Verification items for the finished model (mm, model axes). Coordinates: 2 decimals unless noted, no trailing zeros. Loops run counter-clockwise (first coordinate to the right, second up) from the corner with the lowest first, then second, coordinate; pieces in that order, holes last. Notation, with made-up numbers: (54, -36.5) - (73, -36.5) arc R21 cw to (73, -30.5) - close; hole circle Ø8 at (33.5, 75.5). An arc over 180 degrees is marked (long way). One line per item, written item: value. Start each with the question number.
(1) Section check B-B (y = -33.5). Record the boundary of the cut face in (x, z), plus the area to 3 significant figures.
(2) Section check D-D (z = 34). Record the boundary of the cut face in (x, y).
(3) Section check C-C (x = 2.5). Record the boundary of the cut face in (y, z), plus the area to 3 significant figures.
(4) Thickness scan on probe 1 along Y at (x, z) = (4.3, -25); probe 2 along Y at (x, z) = (4.9, -21.5); probe 3 along Z at (x, y) = (2.5, 9). Record the ranges inside material, lowest first. Write a range as [from, to].
(5) Gauge pin test, flat ends, axial feed: P1, Ø3, axis at x = 4.5, y = -2.5, coming from the +Z side; P2, Ø8, axis at y = -30, z = 50, coming from the -X side. Record the tip position at first contact, or that the pin passes through.
(6) Section check A-A (z = -48). Record the boundary of the cut face in (x, y).
```python
from build123d import *

# Parameters (mm, degrees)
SKETCH1_R           = 5
SKETCH1_R_2         = 2.5
SKETCH1_W           = 10
SKETCH1_H           = 6
SKETCH1_W_2         = 20
BOSS_EXTRUDE1_DEPTH = 6
FILLET1_R           = 5
FILLET2_R           = 1


with BuildPart() as part:
    # Sketch1 → Boss-Extrude1 (new body)
    with BuildSketch(Plane(origin=(0, 0, 0), x_dir=(0, 0, -1), z_dir=(1, 0, 0))):
        with BuildLine():
            Line((0, 5), (65, 5))
            Line((65, 5), (65, 15))
            Line((65, 15), (-35, 15))
            Line((-35, 15), (-62, -21))
            ThreePointArc((-62, -21), (-64.112397745, -35.083328622), (-53.504672381, -44.584830184))
            Line((-53.504672381, -44.584830184), (-6, -56))
            Line((-6, -56), (65, -56))
            Line((65, -56), (65, -44))
            Line((65, -44), (0, -44))
            Line((0, -44), (0, 5))
        make_face()
        with Locations((-50, -30)):
            Circle(SKETCH1_R, mode=Mode.SUBTRACT)
        with Locations((55, 10)):
            Circle(SKETCH1_R_2, mode=Mode.SUBTRACT)
        with Locations((25, 10)):
            Circle(SKETCH1_R_2, mode=Mode.SUBTRACT)
        with Locations((40, -50)):
            Rectangle(SKETCH1_W, SKETCH1_H, mode=Mode.SUBTRACT)
        with Locations((-20, -2)):
            Rectangle(SKETCH1_W_2, SKETCH1_H, mode=Mode.SUBTRACT)
    extrude(amount=BOSS_EXTRUDE1_DEPTH)

    # Fillet1
    fillet1_edges = [part.edges().sort_by_distance(p)[0] for p in [
        (3, -56, -65),
        (3, -56, 6),
        (3, 15, 35),
        (3, 15, -65),
    ]]
    fillet(fillet1_edges, radius=FILLET1_R)

    # Fillet2
    fillet2_edges = [part.edges().sort_by_distance(p)[0] for p in [
        (3, 5, -65),
        (3, -44, -65),
    ]]
    fillet(fillet2_edges, radius=FILLET2_R)


solid = part.part
```
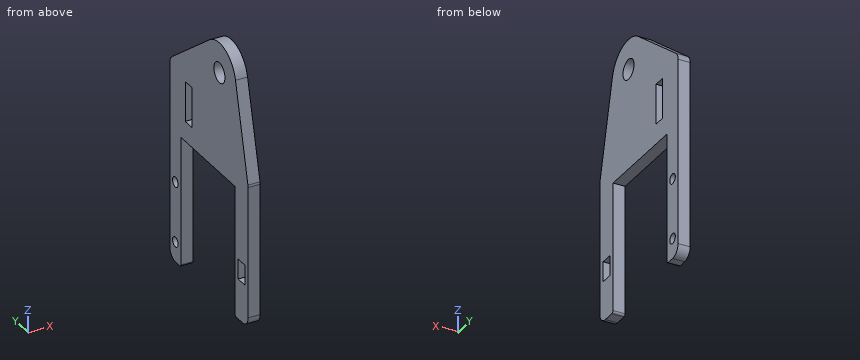
Responses:
1. outline: (0, 0) - (6, 0) - (6, 46.43) - (0, 46.43) - close; (0, 53.57) - (6, 53.57) - (6, 64.59) - (0, 64.59) - close
1. area: 345 mm²
2. outline: (0, -49.27) - (6, -49.27) - (6, 14.77) - (0, 14.77) - close
3. outline: (-56, -60) arc R5 ccw to (-51, -65) - (-45, -65) arc R1 ccw to (-44, -64) - (-44, 0) - (5, 0) - (5, -64) arc R1 ccw to (6, -65) - (10, -65) arc R5 ccw to (15, -60) - (15, 32.5) arc R5 ccw to (13, 36.5) - (-21, 62) arc R15 ccw to (-44.58, 53.5) - (-55.86, 6.58) arc R5 ccw to (-56, 5.41) - close; hole (-53, -45) - (-47, -45) - (-47, -35) - (-53, -35) - close; hole circle Ø10 at (-30, 50); hole (-5, 10) - (1, 10) - (1, 30) - (-5, 30) - close; hole circle Ø5 at (10, -55); hole circle Ø5 at (10, -25)
3. area: 4,690 mm²
4. probe 1: y = [-56, -44], [5, 7.5], [12.5, 15]
4. probe 2: y = [-56, -44], [5, 15]
4. probe 3: z = [-65, -57.29], [-52.71, -27.29], [-22.71, 39.5]
5. P1: stops at z = 49.25
5. P2: passes through
6. outline: (0, -56) - (6, -56) - (6, -44) - (0, -44) - close; (0, 5) - (6, 5) - (6, 15) - (0, 15) - close
